Verification items for this drawing (mm, ordinates from the low corner). A direction names the side the tool comes from. Round coordinates to 2 decimals unless told otherwise and drop trailing zeros. Order: outer loops, then holes, each group sorted by start corner. A loop starts at its lowest first (then second) coordinate and runs counter-clockwise, first axis right, second up. Notation, with made-up numbers: (66, -18.5) - (89, -18.5) arc R14 ccw to (89, -9.5) - close; hole circle Ø10 at (-28, 88.5). An arc over 180 degrees is marked (long way). Use a Markdown table: item, result. Add a question column.
(1) Section check D-D on y = 36. Record the boundary of the cut face in (x, z).
(2) Mould release check, pull along X, two halves, no side actions. Record for the marked faces 3, 4, 5 and 6: released by +X, released by -X, zero draft, split by the parting line, or undercut.
(3) Section check A-A on x = 32.5. Record the boundary of the cut face in (y, z) (1 decimal).
(4) Access from +Z, -Z, +X, -X, +Y, -Y to the whole of each face (thin tool, end or side, straight path). Record for the marked faces 1 and 2.
(5) Thickness scan on line 1 along Y through (x, z) = (35, 4); line 2 along Y through (x, z) = (35, 7); line 3 along Z through (x, y) = (31.5, 66). Record the ranges inside material, lowest first. Write a range as [from, to].
(6) Section check C-C on z = 2.5. Record the boundary of the cut face in (x, y), then the cut area to 3 significant figures.
(7) Gauge pin test, flat ends, axial feed: P1, Ø4, axis at x = 42, y = 10, coming from the +Z side; P2, Ø1, axis at y = 29, z = 3.5, coming from the +X side (3 decimals); P3, Ø6, axis at x = 59.5, z = 5, coming from the -Y side; P4, Ø3, axis at x = 19.5, z = 4.5, coming from the +Y side. Record the tip position at first contact, or that the pin passes through.
(8) Section check B-B on y = 50. Record the boundary of the cut face in (x, z).
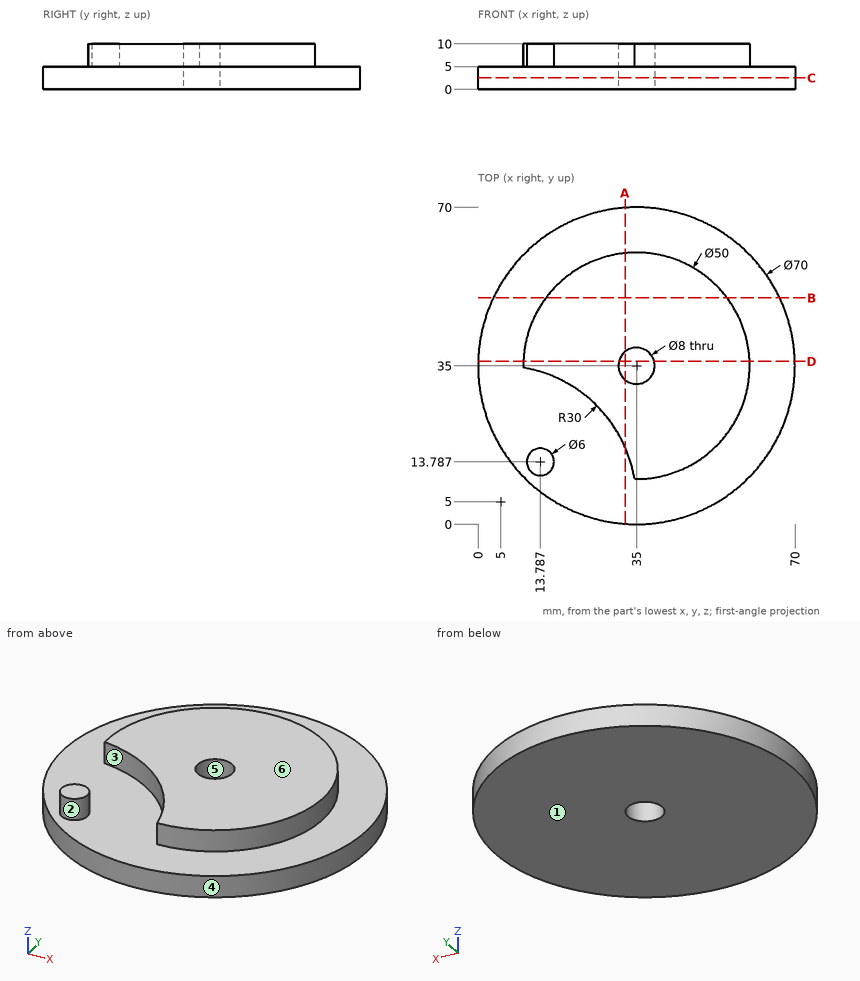
Check sheet entries:
| question | item | result |
|---|---|---|
| 1 | outline | (0.01, 0) - (31.13, 0) - (31.13, 10) - (10.02, 10) - (10.02, 5) - (0.01, 5) - close; (38.87, 0) - (69.99, 0) - (69.99, 5) - (59.98, 5) - (59.98, 10) - (38.87, 10) - close |
| 2 | face 3 | undercut |
| 2 | face 4 | split by the parting line |
| 2 | face 5 | undercut |
| 2 | face 6 | zero draft |
| 3 | outline | (0.1, 0) - (31.9, 0) - (31.9, 10) - (17, 10) - (17, 5) - (0.1, 5) - close; (38.1, 0) - (69.9, 0) - (69.9, 5) - (59.9, 5) - (59.9, 10) - (38.1, 10) - close |
| 4 | face 1 | -Z, +X, -X, +Y, -Y |
| 4 | face 2 | +Z |
| 5 | line 1 | y = [0, 31], [39, 70] |
| 5 | line 2 | y = [10, 31], [39, 60] |
| 5 | line 3 | z = [0, 5] |
| 6 | outline | circle Ø70 at (35, 35); hole circle Ø8 at (35, 35) |
| 6 | area | 3,800 mm2 |
| 7 | P1 | stops at z = 10 |
| 7 | P2 | stops at x = 69.565 |
| 7 | P3 | stops at y = 7.38 |
| 7 | P4 | stops at y = 67.08 |
| 8 | outline | (3.38, 0) - (66.62, 0) - (66.62, 5) - (55, 5) - (55, 10) - (15, 10) - (15, 5) - (3.38, 5) - close |
